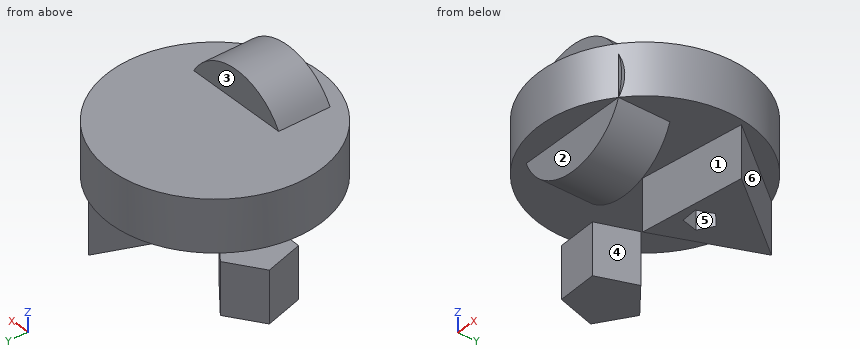
from build123d import *

# Parameters (mm, degrees)
F0_R     = 51.603139
F1_DEPTH = 25.4
F2_R     = 29.816703
F3_DEPTH = 25.4
F5_DEPTH = 25.4


with BuildPart() as f1:
    # F0 (on Top) → F1 (new body)
    with BuildSketch(Plane.XY):
        with Locations((-11.873323, 14.43688)):
            Circle(F0_R)
    extrude(amount=F1_DEPTH)

    # F2 (on Front) → F3 (join)
    with BuildSketch(Plane.XZ):
        with Locations((-7.016055, 10.389157)):
            Circle(F2_R)
    extrude(amount=F3_DEPTH)

    # F4 (on face) → F5 (join)
    with BuildSketch(Plane(origin=(0, 0, 0), x_dir=(1, 0, 0), z_dir=(0, 0, -1))):
        Polygon((-42.001548, -36.874084), (-48.667458, -18.444801), (-68.254628, -19.089496), (-73.694254, -37.917224), (-57.468958, -48.908703), align=None)
        Polygon((5.040846, -63.135175), (36.823419, -22.406714), (-14.339749, -15.246429), align=None)
        Polygon((1.471444, -22.344262), (9.61187, -21.770288), (12.673282, -29.334925), (6.424912, -34.584102), (-0.498204, -30.263635), align=None, mode=Mode.SUBTRACT)
    extrude(amount=F5_DEPTH)


solid = f1.part
Could you check a few things on this model? Use its own coordinates, in mm. Face numbers are marked on the shaded views. A direction names the side the tool comes from. Coordinates: 2 decimals unless noted, no trailing zeros. Order: outer loops, then holes, each group sorted by start corner. A loop starts at its lowest first (then second) coordinate and runs counter-clockwise, first axis right, second up. Notation, with made-up numbers: (89.5, 20.5) -> (141.5, 20.5) arc R14 ccw to (141.5, 34.5) -> close; hole circle Ø5 at (84, 30). An arc over 180 degrees is marked (long way). One line per question, with ' | ' between items.
Q1. Imagine slicing it at C-C on y = -9.5. Please give me the cut outline in (x, z).
Return value:
outline: (-57.59, 0) -> (-34.96, 0) arc R29.82 ccw to (20.93, 0) -> (33.84, 0) -> (33.84, 25.4) -> (18.75, 25.4) arc R29.82 ccw to (-32.78, 25.4) -> (-57.59, 25.4) -> close
Q2. I'm going to push flat-ended pins straight in: P1, Ø6.5, axis at x = 6, y = 29.5, coming from the -Z side; P2, Ø5, axis at y = 21, z = -16, coming from the +X side; P3, Ø3, axis at x = -9.5, z = -3, coming from the +Y side. Where does each tip first touch, or does it pass through?
Return value:
P1: z = 0 | P2: x = 36.82 | P3: y = 30.91
Q3. On a 3-axis mill with a long thin cutter (end or side, diameter ignored), from which of +Z, -Z, +X, -X, +Y, -Y can I reach the whole of each face in a straight line? I mean the marked faces 4, 5 and 6. Say none if no direction works.
Return value:
face 4: -Z, -Y | face 5: -Z | face 6: -Z, +X, +Y
Q4. Imagine slicing it at D-D on z = -15. Please give me the cut outline in (x, y), and give its area (3 significant figures).
Return value:
outline: (-73.69, 37.92) -> (-68.25, 19.09) -> (-48.67, 18.44) -> (-42, 36.87) -> (-57.47, 48.91) -> close; (-22.65, -25.4) -> (8.62, -25.4) -> (8.62, 0) -> (-22.65, 0) -> close; (-14.34, 15.25) -> (36.82, 22.41) -> (5.04, 63.14) -> close; hole (-0.5, 30.26) -> (1.47, 22.34) -> (9.61, 21.77) -> (12.67, 29.33) -> (6.42, 34.58) -> close | area: 2,500 mm²
Q5. Thinking about a two-plate mould opening in Y: for the marked faces 1, 2 and 3, which applies, pulls with the +Y half, pulls with the -Y half, needs draft (parallel to the pull), parting line crosses it, or undercut?
Return value:
face 1: undercut | face 2: pulls with the -Y half | face 3: pulls with the +Y half
Q6. Imagine slicing it at A-A on z = -2.5. Please give me the cut outline in (x, y).
Return value:
outline: (-73.69, 37.92) -> (-68.25, 19.09) -> (-48.67, 18.44) -> (-42, 36.87) -> (-57.47, 48.91) -> close; (-33.9, -25.4) -> (19.87, -25.4) -> (19.87, 0) -> (-33.9, 0) -> close; (-14.34, 15.25) -> (36.82, 22.41) -> (5.04, 63.14) -> close; hole (-0.5, 30.26) -> (1.47, 22.34) -> (9.61, 21.77) -> (12.67, 29.33) -> (6.42, 34.58) -> close
Q7. Imagine slicing it at B-B on x = -21. Please give me the cut outline in (y, z).
Return value:
outline: (-36.35, 0) -> (-25.4, 0) -> (-25.4, -15.94) -> (0, -15.94) -> (0, 0) -> (65.23, 0) -> (65.23, 25.4) -> (0, 25.4) -> (0, 36.72) -> (-25.4, 36.72) -> (-25.4, 25.4) -> (-36.35, 25.4) -> close
Q8. If I drill on L1, parallel to Z at x = -1.5, y = 53.5; L2, parallel to X at y = 15, z = 2; L3, parallel to Z at x = -57, y = 41, over which ranges is the centre line in solid material (lowest first)?
Return value:
L1: 0 to 25.4 | L2: -63.47 to 39.73 | L3: -25.4 to 0
